Work out the finished part from the listing and answer in its coordinate system (mm). Coordinates: 2 decimals unless noted, no trailing zeros. Loops run counter-clockwise (first coordinate to the right, second up) from the corner with the lowest first, then second, coordinate; pieces in that order, holes last. Notation, with made-up numbers: (44, -19) -> (88, -19) arc R19 ccw to (88, -14) -> close; hole circle Ø1 at (-38, 88). An arc over 180 degrees is marked (long way). Use a Markdown table: item, result. Add a question column.
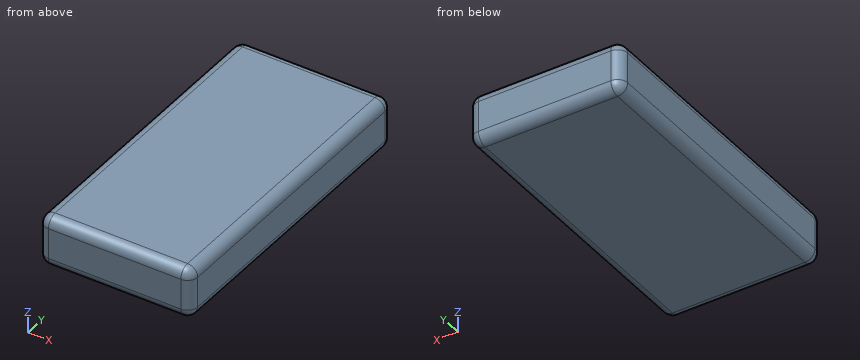
```python
from build123d import *

# Parameters (mm, degrees)
BOX003_W     = 75
BOX003_H     = 150
BOX003_DEPTH = 25
FILLET_R     = 5
FILLET001_R  = 5
FILLET002_R  = 5
FILLET003_R  = 5
FILLET004_R  = 5
FILLET005_R  = 5


with BuildPart() as part:
    # Box003 → Box003 (new body)
    with BuildSketch(Plane(origin=(-37.5, -101, -29), x_dir=(1, 0, 0), z_dir=(0, 0, 1))):
        with Locations((37.5, 75)):
            Rectangle(BOX003_W, BOX003_H)
    extrude(amount=BOX003_DEPTH)

    # Fillet
    fillet_edges = [part.edges().sort_by_distance(p)[0] for p in [
        (-37.5, -26, -4),
    ]]
    fillet(fillet_edges, radius=FILLET_R)

    # Fillet001
    fillet001_edges = [part.edges().sort_by_distance(p)[0] for p in [
        (-37.5, -26, -29),
    ]]
    fillet(fillet001_edges, radius=FILLET001_R)

    # Fillet002
    fillet002_edges = [part.edges().sort_by_distance(p)[0] for p in [
        (37.5, -26, -29),
    ]]
    fillet(fillet002_edges, radius=FILLET002_R)

    # Fillet003
    fillet003_edges = [part.edges().sort_by_distance(p)[0] for p in [
        (37.5, -26, -4),
    ]]
    fillet(fillet003_edges, radius=FILLET003_R)

    # Fillet004
    fillet004_edges = [part.edges().sort_by_distance(p)[0] for p in [
        (0, 49, -29),
    ]]
    fillet(fillet004_edges, radius=FILLET004_R)

    # Fillet005
    fillet005_edges = [part.edges().sort_by_distance(p)[0] for p in [
        (37.5, -101, -16.5),
        (0, -101, -4),
        (0, -101, -29),
        (-37.5, -101, -16.5),
    ]]
    fillet(fillet005_edges, radius=FILLET005_R)


with BuildPart() as part_1:
    # Fillet005 placement: moved
    add(part.part.moved(Location((0, 0, -93.5))))


solid = part_1.part
```
Item 1: Find the intervals of material crossed by probe 1 along X at (y, z) = (38, -102); probe 2 along Y at (x, z) = (33, -113.5); probe 3 along X at (y, z) = (-55.5, -119.75), in increasing order.
Item 2: Section A-A (z = -99.5) is taken. Determine the outline of the cut face in (x, y), then the cut area to 3 significant figures.
Item 3: Given pin 1 (1.5 mm diameter, centred on y = -9, z = -118.5, fed in from +X), flat-ended and moving along its own axis, determine where the tip first touches the part or whether it passes through.
Output:
| question | item | result |
|---|---|---|
| 1 | probe 1 | x = -37.47 to 37.47 |
| 1 | probe 2 | y = -100.97 to 48.97 |
| 1 | probe 3 | x = -36.97 to 36.97 |
| 2 | outline | (-36.5, -96) arc R4 ccw to (-32.5, -100) -> (32.5, -100) arc R4 ccw to (36.5, -96) -> (36.5, 44) arc R4 ccw to (32.5, 48) -> (-32.5, 48) arc R4 ccw to (-36.5, 44) -> close |
| 2 | area | 10,800 mm2 |
| 3 | pin 1 | stops at x = 37.49 |
